```python
from build123d import *

# Parameters (mm, degrees)
F0_W     = 100
F0_H     = 25
F1_DEPTH = 15
F2_W     = 16.6
F2_H     = 6
F3_DEPTH = 73.5
F4_W     = 20
F4_H     = 25
F5_DEPTH = 15
F6_R     = 3.5
F7_DEPTH = 30.001
F8_R     = 3.5
F9_DEPTH = 6


with BuildPart() as f1:
    # F0 (on Top) → F1 (new body)
    with BuildSketch(Plane.XY):
        Rectangle(F0_W, F0_H)
    extrude(amount=F1_DEPTH)

    # F2 (on face) → F3 (cut)
    with BuildSketch(Plane.YZ.offset(50)):
        with Locations((0, 7.786861)):
            Rectangle(F2_W, F2_H)
    extrude(amount=-F3_DEPTH, mode=Mode.SUBTRACT)

    # F4 (on face) → F5 (join)
    with BuildSketch(Plane.XY.offset(15)):
        with Locations((-40, 0)):
            Rectangle(F4_W, F4_H)
    extrude(amount=F5_DEPTH)

    # F6 (on face) → F7 (cut, through all)
    with BuildSketch(Plane.XY.offset(30)):
        with Locations((-40, 0)):
            Circle(F6_R)
    extrude(amount=-F7_DEPTH, mode=Mode.SUBTRACT)

    # F8 (on face) → F9 (cut)
    with BuildSketch(Plane(origin=(0, 0, 0), x_dir=(1, 0, 0), z_dir=(0, 0, -1))):
        Polygon((-40.096797, 6.350115), (-45.54776, 3.091229), (-45.450962, -3.258887), (-39.903203, -6.350115), (-34.45224, -3.091229), (-34.549038, 3.258887), align=None)
        with Locations((-40, 0)):
            Circle(F8_R, mode=Mode.SUBTRACT)
    extrude(amount=-F9_DEPTH, mode=Mode.SUBTRACT)


solid = f1.part
```
Can you work these out from the model? Positions are in its coordinate system, mm. A direction names the side the tool comes from. Give positions to 0.01 mm unless a question says otherwise; leave off trailing zeros. Order: outer loops, then holes, each group sorted by start corner. A loop starts at its lowest first (then second) coordinate and runs counter-clockwise, first axis right, second up. Notation, with made-up numbers: (-28.5, -37.75) - (-11.5, -37.75) arc R27 ccw to (-11.5, -21.75) - close; hole circle Ø4 at (-35.5, 59). An arc over 180 degrees is marked (long way). Use a Markdown table: item, result. Add a question column.
Q1. I'm going to push flat-ended pins straight in: pin 1 (10 mm diameter, centred on y = -4, z = 16, fed in from +X); pin 2 (12 mm diameter, centred on y = -1, z = 21.5, fed in from +X); pin 3 (12.5 mm diameter, centred on x = 6, y = 6, fed in from +Z); pin 4 (3.5 mm diameter, centred on x = -41.5, y = -2.5, fed in from -Z). Where does each tip first touch, or does it pass through?
Q2. If we section it at A-A on x = 28.5: Write out the boundary of the cut face in (y, z), plus the area to 3 significant figures.
Q3. If we mould it in two halves opening along X, with no side actions, what happens to faces 1 (the flat face through (-37.28, -4.78, 2.96)), 2 (the flat face through (-30, 0, 22)), 3 (the flat face through (-42.4, 3, 30))? For each: released by +X, released by -X, zero draft, split by the parting line, or undercut.
Q4. If we section it at C-C on y = 1.5: Write out the boundary of the cut face in (x, z).
Q5. On a 3-axis mill with a long thin cutter (end or side, diameter ignored), from which of +Z, -Z, +X, -X, +Y, -Y can I reach the whole of each face in a straight line? I mean faces 4 (the flat face through (14, 0, 10.787)), 5 (the flat face through (9, 0, 15)), 6 (the flat face through (-42.784, -4.743, 2.958)). Say none if no direction works.
Q6. If we section it at D-D on y = -10: Write out the boundary of the cut face in (x, z).
Q7. If we section it at B-B on z = 11.75: Write out the boundary of the cut face in (x, y), plus the area to 3 significant figures.
Q8. Please list where these lines run through material, in increasing order: line 1 along Z through (x, y) = (35, 3.5); line 2 along X through (y, z) = (0, 19.25); line 3 along Y through (x, z) = (-40, 13.75).
Answers follow:
| question | item | result |
|---|---|---|
| 1 | pin 1 | stops at x = 50 |
| 1 | pin 2 | stops at x = -30 |
| 1 | pin 3 | stops at z = 15 |
| 1 | pin 4 | stops at z = 6 |
| 2 | outline | (-12.5, 0) - (12.5, 0) - (12.5, 15) - (-12.5, 15) - close; hole (-8.3, 4.79) - (8.3, 4.79) - (8.3, 10.79) - (-8.3, 10.79) - close |
| 2 | area | 275 mm^2 |
| 3 | face 1 | undercut |
| 3 | face 2 | released by +X |
| 3 | face 3 | zero draft |
| 4 | outline | (-50, 0) - (-45.48, 0) - (-45.48, 6) - (-43.16, 6) - (-43.16, 30) - (-50, 30) - close; (-36.84, 6) - (-34.48, 6) - (-34.48, 0) - (50, 0) - (50, 4.79) - (-23.5, 4.79) - (-23.5, 10.79) - (50, 10.79) - (50, 15) - (-30, 15) - (-30, 30) - (-36.84, 30) - close |
| 5 | face 4 | +X |
| 5 | face 5 | +Z, +X, +Y, -Y |
| 5 | face 6 | -Z |
| 6 | outline | (-50, 0) - (50, 0) - (50, 15) - (-30, 15) - (-30, 30) - (-50, 30) - close |
| 7 | outline | (-50, -12.5) - (50, -12.5) - (50, 12.5) - (-50, 12.5) - close; hole circle Ø7 at (-40, 0) |
| 7 | area | 2,460 mm^2 |
| 8 | line 1 | z = 0 to 4.79, 10.79 to 15 |
| 8 | line 2 | x = -50 to -43.5, -36.5 to -30 |
| 8 | line 3 | y = -12.5 to -3.5, 3.5 to 12.5 |
